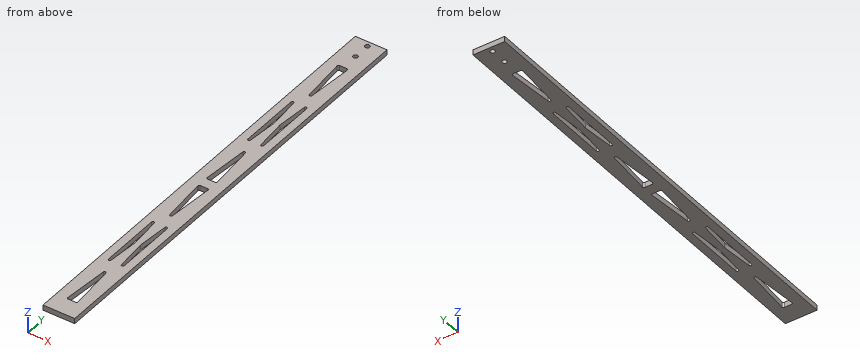
```python
from build123d import *

# Parameters (mm, degrees)
SKETCH1_W           = 38.1
SKETCH1_H           = 533.4
BOSS_EXTRUDE1_DEPTH = 3.175
SKETCH2_R           = 2.778125
CUT_EXTRUDE1_DEPTH  = 294.271022264
CUT_EXTRUDE2_DEPTH  = 294.271022264
FILLET1_R           = 1.5875


with BuildPart() as part:
    # Sketch1 → Boss-Extrude1 (new, symmetric)
    with BuildSketch(Plane.XY):
        with Locations((-6.35, -25.4)):
            Rectangle(SKETCH1_W, SKETCH1_H)
    extrude(amount=BOSS_EXTRUDE1_DEPTH, both=True)

    # Sketch2 → Cut-Extrude1 (cut, through all)
    with BuildSketch(Plane.XY.offset(3.175)):
        with Locations((-6.35, 234.95)):
            Circle(SKETCH2_R)
        with Locations((-6.35, 214.63)):
            Circle(SKETCH2_R)
    extrude(amount=-CUT_EXTRUDE1_DEPTH, mode=Mode.SUBTRACT)

    # Sketch3 → Cut-Extrude2 (cut, through all)
    with BuildSketch(Plane.XY.offset(3.175)):
        Polygon((-6.291879002, 118.898888525), (-0.011179953, 193.675), (-12.57257805, 193.675), align=None)
        Polygon((3.175, 6.189078026), (3.175, 155.741300976), (-3.105699049, 80.965189501), align=None)
        Polygon((-15.758758004, 6.189078026), (-9.478058955, 80.965189501), (-15.758758004, 155.741300976), align=None)
        Polygon((-0.011179953, -31.744620998), (-6.291879002, 43.031490477), (-12.57257805, -31.744620998), align=None)
        Polygon((-6.291879002, -119.220732473), (-0.011179953, -44.444620998), (-12.57257805, -44.444620998), align=None)
        Polygon((3.175, -231.930542972), (3.175, -82.378320022), (-3.105699049, -157.154431497), align=None)
        Polygon((-9.478058955, -157.154431497), (-15.758758004, -82.378320022), (-15.758758004, -231.930542972), align=None)
        Polygon((-0.011179953, -269.864241996), (-6.291879002, -195.088130521), (-12.57257805, -269.864241996), align=None)
    extrude(amount=-CUT_EXTRUDE2_DEPTH, mode=Mode.SUBTRACT)

    # Fillet1
    fillet1_edges = [part.edges().sort_by_distance(p)[0] for p in [
        (-6.291879002, -119.220732473, 0),
        (-12.57257805, -44.444620998, 0),
        (-0.011179953, -44.444620998, 0),
        (-6.291879002, 43.031490477, 0),
        (-0.011179953, -31.744620998, 0),
        (-12.57257805, -31.744620998, 0),
        (-15.758758004, 155.741300976, 0),
        (-9.478058955, 80.965189501, 0),
        (-15.758758004, 6.189078026, 0),
        (-3.105699049, 80.965189501, 0),
        (3.175, 155.741300976, 0),
        (3.175, 6.189078026, 0),
        (-12.57257805, -269.864241996, 0),
        (-6.291879002, -195.088130521, 0),
        (-0.011179953, -269.864241996, 0),
        (-15.758758004, -231.930542972, 0),
        (-15.758758004, -82.378320022, 0),
        (-9.478058955, -157.154431497, 0),
        (-3.105699049, -157.154431497, 0),
        (3.175, -82.378320022, 0),
        (3.175, -231.930542972, 0),
        (-12.57257805, 193.675, 0),
        (-0.011179953, 193.675, 0),
        (-6.291879002, 118.898888525, 0),
    ]]
    fillet(fillet1_edges, radius=FILLET1_R)


solid = part.part
```
CAD build for the part. Positions are in the model's coordinates, mm. Round coordinates to 2 decimals unless told otherwise and drop trailing zeros. Order: outer loops, then holes, each group sorted by start corner. A loop starts at its lowest first (then second) coordinate and runs counter-clockwise, first axis right, second up. Notation, with made-up numbers: (32.5, 60) -> (76.5, 60) arc R27 ccw to (76.5, 87) -> close; hole circle Ø8 at (37, 56). An arc over 180 degrees is marked (long way). Write item = value, one per line.
(1) Cut at C-C (y = -234). Write the cut outline in (x, z) (3 decimals).
Answers follow:
outline = (-25.4, -3.175) -> (-9.56, -3.175) -> (-9.56, 3.175) -> (-25.4, 3.175) -> close; (-3.024, -3.175) -> (12.7, -3.175) -> (12.7, 3.175) -> (-3.024, 3.175) -> close
(2) Flat gauge pin, fed straight in: P1, Ø4.5, axis at x = -6.35, y = 214.63, coming from the +Z side. Where does the tip first touch, or does it go through?
Answers follow:
P1 = through
(3) Drill centre lines: L1, parallel to Y at x = 2, z = -2.5; L2, parallel to X at y = 214.63, z = 1.25; L3, parallel to X at y = -182.5, z = -1.5 (3 decimals). Where is each one in solid material? Low to high.
Answers follow:
L1 = -292.1 to -195.6, -118.71 to 42.52, 119.41 to 241.3
L2 = -25.4 to -9.13, -3.57 to 12.7
L3 = -25.4 to -15.759, -11.607 to -0.977, 3.175 to 12.7
(4) Cut at A-A (y = -25). Write the cut outline in (x, z) (3 decimals), plus the area to 3 significant figures.
Answers follow:
outline = (-25.4, -3.175) -> (-12.006, -3.175) -> (-12.006, 3.175) -> (-25.4, 3.175) -> close; (-0.578, -3.175) -> (12.7, -3.175) -> (12.7, 3.175) -> (-0.578, 3.175) -> close
area = 169 mm²
(5) Cut at B-B (z = -0.5). State how many separate pieces and enclosed holes the cut face has, plus the area to 3 significant figures.
Answers follow:
separate_pieces = 1
enclosed_holes = 10
area = 17,100 mm²
